Autodesk Inventor part; units mm, degrees
ref_plane "YZ Plane" through (0, 0, 0) normal (1, 0, 0) x (0, 1, 0)
ref_plane "XZ Plane" through (0, 0, 0) normal (0, 1, 0) x (-1, 0, 0)
ref_plane "XY Plane" through (0, 0, 0) normal (0, 0, 1) x (1, 0, 0)
sketch "草图1" plane through (0, 0, 0) normal (0, 0, 1) x (1, 0, 0)
  circle A0 centre (0, 0) radius 2
  dimension "d0" = 4
extrude "拉伸1" add sketch "草图1" along normal blind 15
sketch "草图2" plane through (0, 0, 15) normal (0, 0, 1) x (1, 0, 0)
  line L0 (-0.75, 2) -> (0.75, 2)
  line L1 (0.75, 2) -> (0.75, -2)
  line L2 (0.75, -2) -> (-0.75, -2)
  line L3 (-0.75, -2) -> (-0.75, 2)
  line L4 (0, 0) -> (0, 2)
  circle A0 centre (0, 0) radius 2
  dimension "d3" = 1.5
extrude "拉伸2" cut sketch "草图2" against normal blind 3 contours L0 A0 L3 | L0 L1 A0 | A0 L1 L3 | A0 L2 L3 | L1 L2 A0
thread "螺纹1"
chamfer "倒角1" distance 0.25 angle 45 1 edges at (-2, 0, 0)
properties part number "砂轮电机皮带轮固定螺丝"
The model under review builds one solid part; all positions refer to its coordinate system, in mm. A direction names the side the tool comes from. Coordinates: 2 decimals unless noted, no trailing zeros. Write each loop counter-clockwise with the first axis right and the second up, starting at its lowest first coordinate (ties: lowest second). Pieces come first, ordered by that corner, then holes. Notation, with made-up numbers: (23.25, 62.5) - (42.25, 62.5) arc R12 ccw to (42.25, 80.5) - close; hole circle Ø9 at (87.5, 43). An arc over 180 degrees is marked (long way). Answer in a Markdown table with one row per item. Add a question column.
Q1. Draft analysis for pull direction X (two halves, no side actions). For faces 1 (the face through (1, 0, 15)), 2 (the face through (1.847, 0.766, 7.522)), 3 (the face through (0.75, 0, 14)), state which applies: +X half, -X half, draft (parallel to the pull), parting line (faces both ways), or undercut.
Q2. Consider section D-D on z = 7. Give the boundary of the cut face in (x, y).
Q3. Consider section A-A on y = 0. Give the boundary of the cut face in (x, z), then the cut area to 3 significant figures.
Q4. Consider section C-C on z = 13.5. Give the boundary of the cut face in (x, y).
Q5. Clearance check with a flat-ended pin moving along its axis: pin 1 (1 mm diameter, centred on x = 0, y = -0.5, fed in from +Z). State where the tip first meets the part, or that it passes through.
Q6. To check wall thickness, follow line 1 along Z through (x, y) = (0, -0.05); line 2 along X through (y, z) = (-0.15, 12.75); line 3 along X through (y, z) = (1.7, 6). State the ranges of each line that lie inside material, in increasing order. Write a range as from..to.
Q7. Consider section B-B on x = 0. Give the boundary of the cut face in (y, z), then the cut area to 3 significant figures.
Q8. For faces 4 (the face through (-0.75, 0, 14)), 5 (the face through (-1, 0, 15)), list the 3-axis set-ups (+Z, -Z, +X, -X, +Y, -Y) from which the entire face can be reached by the end or side of a thin tool; tool diameter is ignored.
Answers below:
| question | item | result |
|---|---|---|
| 1 | face 1 | draft |
| 1 | face 2 | parting line |
| 1 | face 3 | undercut |
| 2 | outline | circle Ø4 at (0, 0) |
| 3 | outline | (-2, 0.25) - (-1.75, 0) - (1.75, 0) - (2, 0.25) - (2, 15) - (0.75, 15) - (0.75, 12) - (-0.75, 12) - (-0.75, 15) - (-2, 15) - close |
| 3 | area | 55.4 mm² |
| 4 | outline | (-0.75, -1.85) - (-0.75, 1.85) arc R2 ccw to start; (0.75, -1.85) arc R2 ccw to (0.75, 1.85) - close |
| 5 | pin 1 | z = 12 |
| 6 | line 1 | 0..12 |
| 6 | line 2 | -1.99..-0.75, 0.75..1.99 |
| 6 | line 3 | -1.05..1.05 |
| 7 | outline | (-2, 0.25) - (-1.75, 0) - (1.75, 0) - (2, 0.25) - (2, 12) - (-2, 12) - close |
| 7 | area | 47.9 mm² |
| 8 | face 4 | +Z, +Y, -Y |
| 8 | face 5 | +Z, +X, -X, +Y, -Y |
